The model under review builds one solid part; all positions refer to its coordinate system, in mm. Face numbers are marked on the shaded views. A direction names the side the tool comes from. Coordinates: 2 decimals unless noted, no trailing zeros. Loops run counter-clockwise (first coordinate to the right, second up) from the corner with the lowest first, then second, coordinate; pieces in that order, holes last. Notation, with made-up numbers: (5, -3.75) - (54, -3.75) arc R19 ccw to (54, 3.25) - close; hole circle Ø3 at (33, -1.75). An arc over 180 degrees is marked (long way). Use a Markdown table: item, result. Add a question column.
1) Clearance check with flat-ended pins moving along their axes: pin 1 (2.5 mm diameter, centred on x = -9, z = -0.5, fed in from +Y); pin 2 (1.5 mm diameter, centred on x = -2.5, z = -1, fed in from -Y); pin 3 (1.6 mm diameter, centred on x = 0, y = 0, fed in from -Z); pin 4 (1.5 mm diameter, centred on y = -2, z = -1.5, fed in from +X). State where each tip first meets the part, or that it passes through.
2) To check wall thickness, follow L1, parallel to Y at x = 12, z = -1.3; L2, parallel to Z at x = 5.5, y = 16.5; L3, parallel to X at y = -0.5, z = -4.9. State the ranges of each line that lie inside material, in increasing order. Write a range as [from, to].
3) Add section D-D, the plane y = 0. Give the number of separate pieces and of enclosed holes in the cut face, and give its area (3 significant figures).
4) The part is to be moulded in two halves that separate along Y. For the marked faces 1, 2 and 3, say which applies: pulls with the +Y half, pulls with the -Y half, needs draft (parallel to the pull), parting line crosses it, or undercut.
5) Add section A-A, the plane x = -12. Give the boundary of the cut face in (y, z), and give its area (4 significant figures).
6) Add section B-B, the plane y = 10. Give the boundary of the cut face in (x, z).
7) Add section C-C, the plane z = -4.75. Give the boundary of the cut face in (x, y).
8) For the marked faces 4, 5, 6, 7 and 8, list the 3-axis set-ups (+Z, -Z, +X, -X, +Y, -Y) from which the entire face can be reached by the end or side of a thin tool; tool diameter is ignored.
Autodesk Inventor part; units mm, degrees
ref_plane "YZ Plane" through (0, 0, 0) normal (1, 0, 0) x (0, 1, 0)
ref_plane "XZ Plane" through (0, 0, 0) normal (0, 1, 0) x (-1, 0, 0)
ref_plane "XY Plane" through (0, 0, 0) normal (0, 0, 1) x (1, 0, 0)
sketch "Sketch1" plane through (0, 0, 0) normal (0, 0, 1) x (1, 0, 0)
  arc A0 (6, 16) -> (-6, 16) centre (0, 16) ccw
  line L0 (0, -30.8) -> (0, 30.8) construction
  line L1 (-6, 16) -> (-6, 6)
  line L2 (6, 16) -> (6, 6)
  circle A1 centre (0, 13) radius 0.75
  circle A2 centre (0, 10) radius 0.75
  circle A3 centre (0, 19) radius 0.75
  circle A4 centre (0, 16) radius 0.75
  line L3 (-7.8151, 0) -> (8.8196, 0) construction
  arc A5 (-6, -16) -> (6, -16) centre (0, -16) ccw
  line L4 (-6, -16) -> (-6, -6)
  line L5 (6, -16) -> (6, -6)
  circle A6 centre (0, -13) radius 0.75
  circle A7 centre (0, -10) radius 0.75
  circle A8 centre (0, -19) radius 0.75
  circle A9 centre (0, -16) radius 0.75
  line L6 (6, 6) -> (15, 6)
  arc A10 (15, -6) -> (15, 6) centre (15, 0) ccw
  line L7 (15, 6) -> (15, -6) construction
  line L8 (15, 6) -> (27, 6) construction
  line L9 (15, -6) -> (6, -6)
  circle A11 centre (18, 0) radius 0.75
  circle A12 centre (15, 0) radius 0.75
  circle A13 centre (12, 0) radius 0.75
  line L10 (7.8151, 0) -> (-8.8196, 0) construction
  line L11 (-6, 6) -> (-15, 6)
  arc A14 (-15, 6) -> (-15, -6) centre (-15, 0) ccw
  line L12 (-15, 6) -> (-15, -6) construction
  line L13 (-15, -6) -> (-6, -6)
  circle A15 centre (-18, 0) radius 0.75
  circle A16 centre (-15, 0) radius 0.75
  circle A17 centre (-12, 0) radius 0.75
  line L14 (6, 6) -> (6, -6)
  line L15 (-6, 6) -> (-6, -6)
  point P0 (0, 0)
  dimension "d0" = 12
  dimension "d1" = 6
  dimension "d2" = 10
  dimension "d3" = 10
  dimension "d5" = 1.5
  dimension "d6" = 1.5
  dimension "d8" = 1.5
  dimension "d9" = 13
  dimension "d10" = 10
  dimension "d11" = 19
  dimension "d12" = 1.5
  dimension "d13" = 16
  dimension "d14" = 16
  dimension "d15" = 10
  dimension "d16" = 90
  dimension "d17" = 6
  dimension "d18" = 15
  dimension "d19" = 12
  dimension "d20" = 15
  dimension "d21" = 18
  dimension "d22" = 1.5
  dimension "d23" = 1.5
  dimension "d24" = 1.5
  dimension "d25" = 6
  dimension "d26" = 6
extrude "Extrusion1" add sketch "Sketch1" against normal blind 3 contours L2 L14 L5 A5 L4 L15 L1 A0
extrude "Extrusion2" add sketch "Sketch1" against normal blind 2.1 contours L6 A10 L9 L14 | L15 L13 A14 L11
sketch "Sketch2" plane through (0, 0, -3) normal (0, 0, -1) x (-1, 0, 0)
  circle A0 centre (0, 0) radius 5
  dimension "d31" = 10
extrude "Extrusion3" add sketch "Sketch2" along normal blind 2.85
sketch "Sketch3" plane through (0, 0, -5.85) normal (0, 0, -1) x (-1, 0, 0)
  point P0 (0, 0)
  point P1 (0, 0)
hole "Hole1" at (0, 0, -5.85) direction (0, 0, 1) diameter 5.5 depth 2.85
sketch "Sketch6" plane through (0, 0, 0) normal (0, 0, 1) x (1, 0, 0)
  point P0 (0, 0)
  point P1 (0, 0)
hole "Hole2" at (0, 0, 0) direction (0, 0, -1) diameter 6 depth 1.4
sketch "Sketch7" plane through (0, 0, -1.4) normal (0, 0, 1) x (1, 0, 0)
  point P0 (0, 0)
  point P1 (0, 0)
hole "Hole3" at (0, 0, -1.4) direction (0, 0, -1) diameter 2.7 end through all
equation "\"d2\" = d3"
equation "\"d5\" = d8"
equation "\"d6\" = d8"
equation "\"d12\" = d8"
equation "\"d22\" = d8"
equation "\"d23\" = d8"
equation "\"d24\" = d8"
properties part number "Servo Horn 3 Skiba"
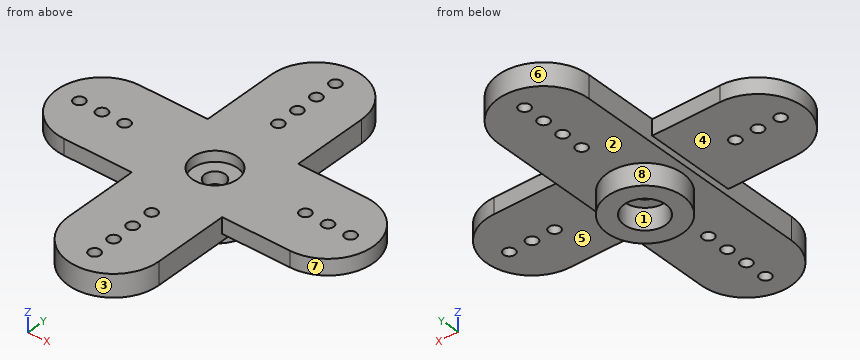
From the geometry:
| question | item | result |
|---|---|---|
| 1 | pin 1 | stops at y = 6 |
| 1 | pin 2 | stops at y = -21.74 |
| 1 | pin 3 | passes through |
| 1 | pin 4 | stops at x = 20.87 |
| 2 | L1 | y = [-6, -0.75], [0.75, 6] |
| 2 | L2 | z = [-3, 0] |
| 2 | L3 | x = [-4.97, -2.7], [2.7, 4.97] |
| 3 | separate pieces | 8 |
| 3 | enclosed holes | 0 |
| 3 | area | 80.2 mm^2 |
| 4 | face 1 | undercut |
| 4 | face 2 | needs draft |
| 4 | face 3 | pulls with the -Y half |
| 5 | outline | (-6, -2.1) - (-0.75, -2.1) - (-0.75, 0) - (-6, 0) - close; (0.75, -2.1) - (6, -2.1) - (6, 0) - (0.75, 0) - close |
| 5 | area | 22.05 mm^2 |
| 6 | outline | (-6, -3) - (-0.75, -3) - (-0.75, 0) - (-6, 0) - close; (0.75, -3) - (6, -3) - (6, 0) - (0.75, 0) - close |
| 7 | outline | circle Ø10 at (0, 0); hole circle Ø5.5 at (0, 0) |
| 8 | face 4 | -Z, -X, +Y, -Y |
| 8 | face 5 | -Z, +X, +Y, -Y |
| 8 | face 6 | +Z, -Z, +Y |
| 8 | face 7 | +Z, -Z, +X |
| 8 | face 8 | -Z |
